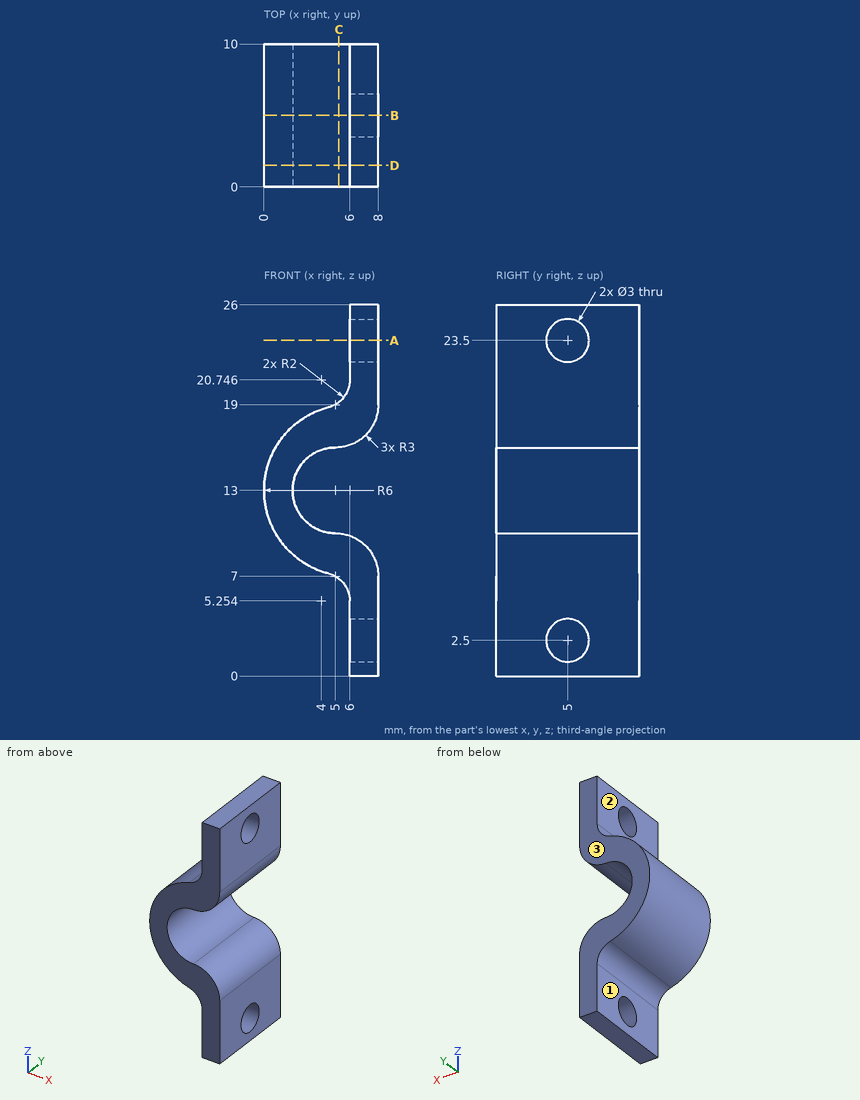
The drawing under review shows one solid part. Ordinate dimensions are in mm from its lowest x, y, z. A direction names the side the tool comes from. Round coordinates to 2 decimals unless told otherwise and drop trailing zeros. Write each loop counter-clockwise with the first axis right and the second up, starting at its lowest first coordinate (ties: lowest second). Pieces come first, ordered by that corner, then holes. Notation, with made-up numbers: (21, 21) - (26, 21) arc R20 cw to (26, 33) - close; hole circle Ø3 at (-19, 59). An arc over 180 degrees is marked (long way). Use one line per item in the form item = value.
Q1. Consider section B-B (y = 5). State the section outline as (x, z) points, and give its area (3 significant figures).
Answer key:
outline = (4.5, 7.19) arc R2 cw to (6, 5.25) - (6, 4) - (8, 4) - (8, 7) arc R3 ccw to (5, 10) arc R3 cw to (5, 16) arc R3 ccw to (8, 19) - (8, 22) - (6, 22) - (6, 20.75) arc R2 cw to (4.5, 18.81) arc R6 ccw to start; (6, 0) - (8, 0) - (8, 1) - (6, 1) - close; (6, 25) - (8, 25) - (8, 26) - (6, 26) - close
area = 61.7 mm2
Q2. Consider section D-D (y = 1.5). State the section outline as (x, z) points, and give its area (3 significant figures).
Answer key:
outline = (4.5, 7.19) arc R2 cw to (6, 5.25) - (6, 0) - (8, 0) - (8, 7) arc R3 ccw to (5, 10) arc R3 cw to (5, 16) arc R3 ccw to (8, 19) - (8, 26) - (6, 26) - (6, 20.75) arc R2 cw to (4.5, 18.81) arc R6 ccw to start
area = 73.7 mm2
Q3. Consider section A-A (z = 23.5). State the section outline as (x, y) points, and give its area (3 significant figures).
Answer key:
outline = (6, 0) - (8, 0) - (8, 3.5) - (6, 3.5) - close; (6, 6.5) - (8, 6.5) - (8, 10) - (6, 10) - close
area = 14.0 mm2
Q4. Consider section C-C (x = 5.25). State the section outline as (y, z) points, and give its area (3 significant figures).
Answer key:
outline = (0, 6.82) - (10, 6.82) - (10, 9.99) - (0, 9.99) - close; (0, 16.01) - (10, 16.01) - (10, 19.18) - (0, 19.18) - close
area = 63.5 mm2
Q5. For line 1 (Y direction, x = 6.4, z = 2.5); line 2 (Z direction, x = 7, y = 5); line 3 (Z direction, x = 6.95, y = 5), list the stretches that pass through material, from the lowest coordinate up. Write a range as [from, to].
Answer key:
line_1 = [0, 3.5], [6.5, 10]
line_2 = [0, 1], [4, 9.24], [16.76, 22], [25, 26]
line_3 = [0, 1], [4, 9.28], [16.72, 22], [25, 26]
Q6. Tool access review of the marked faces 1, 2 and 3: name each direction out of +Z, -Z, +X, -X, +Y, -Y from which nothing blocks a thin tool from reaching the whole face with its end or side.
Answer key:
face_1 = -Z, -X, +Y, -Y
face_2 = +Z, -X, +Y, -Y
face_3 = +Z, -Z, +X, -X, +Y
Q7. Insertion check: pin 1 Ø5 at (y, z) = (5, 16) entering from +X; pin 2 Ø4 at (x, y) = (2.5, 7.5) entering from +Z; pin 3 Ø2.5 at (y, z) = (3.5, 2) entering from -X. Each pin has a flat end and moves straight along its axis. Give the tip position at first contact, or say it passes through.
Answer key:
pin_1 = 7.96
pin_2 = 18.81
pin_3 = 6
